Can you work these out from the model? Positions are in its coordinate system, mm. A direction names the side the tool comes from. Give positions to 0.01 mm unless a question says otherwise; leave off trailing zeros. Loops run counter-clockwise (first coordinate to the right, second up) from the corner with the lowest first, then second, coordinate; pieces in that order, holes last. Notation, with made-up numbers: M 35,1.25 L 39,1.25 A24 cw 39,16.25 Z; hole C -24,81.25 d7. An arc over 180 degrees is marked long. Put each result on its own line as item: value. Start each with the question number.
1) Imagine slicing it at B-B (x = -13). Write out the boundary of the cut face in (y, z), then the cut area to 3 significant figures.
2) Imagine slicing it at C-C (z = 5.25). Write out the boundary of the cut face in (x, y), then the cut area to 3 significant figures.
3) Imagine slicing it at A-A (y = -10.75). Write out the boundary of the cut face in (x, z), then the cut area to 3 significant figures.
4) For faces 4 (the flat face through (-8.1, -6, 12)), 5 (the flat face through (-10.6, 0, 0)), 6 (the flat face through (8.1, 6, 12)), 7 (the flat face through (8.1, -6, -12)), 8 (the flat face through (-8.1, -6, -12)), which set-ups out of +Z, -Z, +X, -X, +Y, -Y let a thin tool reach every point of the face, with its end or its side?
5) Imagine slicing it at D-D (x = 10). Write out the boundary of the cut face in (y, z).
6) If we mould it in two halves opening along Z, with no side actions, what happens to faces 1 (the flat face through (0, -6, -14.5)), 2 (the flat face through (0, -8, -8.5)), 3 (the flat face through (0, 5.1, 3))? For each: +Z half, -Z half, draft (parallel to the pull), parting line (faces both ways), or undercut.
7) Please list where these lines run through material, in increasing order: line 1 along X through (y, z) = (4, 8); line 2 along Y through (x, z) = (4.5, -2.75); line 3 along Z through (x, y) = (-13.5, 10.75). Write a range as from..to.
8) For P1, Ø3, axis at y = -4, z = -3.5, coming from the -X side; P2, Ø1.5, axis at x = -2.5, z = 13, coming from the -Y side; P3, Ø10, axis at x = 2, y = -3, coming from the -Z side; P4, Ø1.5, axis at x = 1, z = 12.5, coming from the +Y side, each with a flat end and sliding along its axis, tell me the tip position at first contact or that it passes through.
from build123d import *

# Parameters (mm, degrees)
BOSS_EXTRUDE1_DEPTH      = 9.5
BOSS_EXTRUDE1_DEPTH_BACK = 9.5
SKETCH1_W                = 31.2
SKETCH1_H                = 25.2
SKETCH1_W_2              = 16.2
SKETCH1_H_2              = 10.2
SKETCH2_W                = 31.2
SKETCH2_H                = 17
CUT_EXTRUDE1_DEPTH       = 5
SKETCH3_W                = 17
SKETCH3_H                = 15.2
CUT_EXTRUDE2_DEPTH       = 5
SKETCH4_W                = 16.2
SKETCH4_H                = 2
BOSS_EXTRUDE2_DEPTH      = 5
SKETCH6_W                = 16.2
SKETCH6_H                = 5
CUT_EXTRUDE3_DEPTH       = 2


with BuildPart() as part:
    # Sketch1 → Boss-Extrude1 (new, two sides: drawn at the far end of the back side and taken through both)
    with BuildSketch(Plane.XY.offset(-BOSS_EXTRUDE1_DEPTH_BACK)):
        Rectangle(SKETCH1_W, SKETCH1_H)
        Rectangle(SKETCH1_W_2, SKETCH1_H_2, mode=Mode.SUBTRACT)
    extrude(amount=BOSS_EXTRUDE1_DEPTH + BOSS_EXTRUDE1_DEPTH_BACK)

    # Sketch2 → Cut-Extrude1 (cut)
    with BuildSketch(Plane(origin=(0, 12.6, 0), x_dir=(1, 0, 0), z_dir=(0, 1, 0))):
        Rectangle(SKETCH2_W, SKETCH2_H)
    cut_extrude1 = extrude(amount=-CUT_EXTRUDE1_DEPTH, mode=Mode.SUBTRACT)

    # Mirror1: Cut-Extrude1 across plane
    add(cut_extrude1.mirror(Plane.ZX), mode=Mode.SUBTRACT)

    # Sketch3 → Cut-Extrude2 (cut)
    with BuildSketch(Plane(origin=(15.6, 0, 0), x_dir=(0, 0, -1), z_dir=(1, 0, 0))):
        Rectangle(SKETCH3_W, SKETCH3_H)
    cut_extrude2 = extrude(amount=-CUT_EXTRUDE2_DEPTH, mode=Mode.SUBTRACT)

    # Mirror2: Cut-Extrude2 across plane
    add(cut_extrude2.mirror(Plane(origin=(0, 0, 0), x_dir=(0, 0, 1), z_dir=(1, 0, 0))), mode=Mode.SUBTRACT)

    # Sketch4 → Boss-Extrude2 (add)
    with BuildSketch(Plane.XY.offset(9.5)):
        with Locations((0, 6.1)):
            Rectangle(SKETCH4_W, SKETCH4_H)
        with Locations((0, -6.1)):
            Rectangle(SKETCH4_W, SKETCH4_H)
    boss_extrude2 = extrude(amount=BOSS_EXTRUDE2_DEPTH)

    # Mirror3: Boss-Extrude2 across plane
    add(boss_extrude2.mirror(Plane.XY))

    # Sketch6 → Cut-Extrude3 (cut)
    with BuildSketch(Plane(origin=(0, 7.1, 0), x_dir=(1, 0, 0), z_dir=(0, 1, 0))):
        with Locations((0, 12)):
            Rectangle(SKETCH6_W, SKETCH6_H)
    extrude(amount=-CUT_EXTRUDE3_DEPTH, mode=Mode.SUBTRACT)


solid = part.part
Recorded:
1. outline: M -12.6,-9.5 L 12.6,-9.5 L 12.6,-8.5 L -12.6,-8.5 Z; M -12.6,8.5 L 12.6,8.5 L 12.6,9.5 L -12.6,9.5 Z
1. area: 50.4 mm²
2. outline: M -10.6,-7.6 L 10.6,-7.6 L 10.6,7.6 L -10.6,7.6 Z; hole M -8.1,-5.1 L 8.1,-5.1 L 8.1,5.1 L -8.1,5.1 Z
2. area: 157 mm²
3. outline: M -15.6,-9.5 L 15.6,-9.5 L 15.6,-8.5 L -15.6,-8.5 Z; M -15.6,8.5 L 15.6,8.5 L 15.6,9.5 L -15.6,9.5 Z
3. area: 62.4 mm²
4. face 4: +Z, -X, +Y, -Y
4. face 5: -X, +Y, -Y
4. face 6: +Z, +X, +Y, -Y
4. face 7: -Z, +X, +Y, -Y
4. face 8: -Z, -X, +Y, -Y
5. outline: M -12.6,-9.5 L 12.6,-9.5 L 12.6,-8.5 L 7.6,-8.5 L 7.6,8.5 L 12.6,8.5 L 12.6,9.5 L -12.6,9.5 L -12.6,8.5 L -7.6,8.5 L -7.6,-8.5 L -12.6,-8.5 Z
6. face 1: -Z half
6. face 2: undercut
6. face 3: draft
7. line 1: -10.6..-8.1, 8.1..10.6
7. line 2: -7.6..-5.1, 5.1..7.6
7. line 3: -9.5..-8.5, 8.5..9.5
8. P1: x = -10.6
8. P2: y = -7.1
8. P3: z = -14.5
8. P4: y = 7.1
